CAD build for the part. Positions are in the model's coordinates, mm. Face numbers are marked on the shaded views. A direction names the side the tool comes from. Round coordinates to 2 decimals unless told otherwise and drop trailing zeros. Loops run counter-clockwise (first coordinate to the right, second up) from the corner with the lowest first, then second, coordinate; pieces in that order, holes last. Notation, with made-up numbers: M -39,-7 L -4,-7 A17 ccw -4,18 Z; hole C -29.5,-38.5 d4. An arc over 180 degrees is marked long. One line per item, written item: value. Start each with the question number.
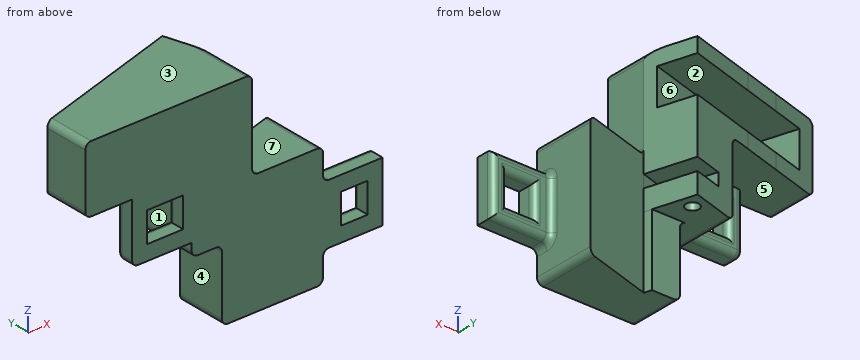
from build123d import *

# Parameters (mm, degrees)
SKETCH2_W                       = 43.976301399
SKETCH2_H                       = 37.406376753
BOSS_EXTRUDE1_DEPTH             = 3
BOSS_EXTRUDE2_REACH             = 40.151
BOSS_EXTRUDE2_DIRECTION_2_REACH = 40.151
SKETCH4_W                       = 23.72463769
SKETCH4_H                       = 6.1
CUT_EXTRUDE1_DEPTH              = 6.2
SKETCH5_W                       = 13.436339427
SKETCH5_H                       = 17.119562917
CUT_EXTRUDE2_DEPTH              = 42.11242086
CUT_EXTRUDE3_DEPTH              = 40.896849069
CUT_EXTRUDE3_DEPTH_BACK         = 40.896849069
SKETCH6_W                       = 32.063710036
SKETCH6_H                       = 2.195719192
SKETCH7_W                       = 17.859472784
SKETCH7_H                       = 24.110657561
CUT_EXTRUDE4_DEPTH              = 39.572188243
SKETCH9_W                       = 5.100000004
SKETCH9_H                       = 2.100000005
CUT_EXTRUDE5_DEPTH              = 8.272220174
SKETCH10_W                      = 4.059731886
SKETCH10_H                      = 35.210657561
CUT_EXTRUDE6_DEPTH              = 39.572188243
CUT_EXTRUDE7_DEPTH              = 11.9
SKETCH14_W                      = 10
SKETCH14_H                      = 3
BOSS_EXTRUDE3_DEPTH             = 10
SKETCH15_W                      = 4.5
SKETCH15_H                      = 5
CUT_EXTRUDE8_DEPTH              = 47.530169979
FILLET1_R                       = 1
CUT_EXTRUDE9_DEPTH              = 49.140668642
CUT_EXTRUDE10_DEPTH             = 11.9
SKETCH19_R                      = 1.1
CUT_EXTRUDE11_DEPTH             = 47.161274086
BOSS_EXTRUDE4_DEPTH             = 11.9
FILLET2_R                       = 1
SKETCH22_W                      = 10
SKETCH22_H                      = 3
BOSS_EXTRUDE5_DEPTH             = 10
SKETCH23_W                      = 6.079403202
SKETCH23_H                      = 5
CUT_EXTRUDE12_DEPTH             = 47.530169979
FILLET4_R                       = 1


with BuildPart() as part:
    # Sketch2 → Boss-Extrude1 (new body)
    with BuildSketch(Plane(origin=(0, 0, 0), x_dir=(1, 0, 0), z_dir=(0, 1, 0))):
        with Locations((6.873999922, -6.064560357)):
            Rectangle(SKETCH2_W, SKETCH2_H)
    extrude(amount=BOSS_EXTRUDE1_DEPTH)

    # Boss-Extrude2: up to this face of the body (flat: up to its plane)
    boss_extrude2_end = Plane(part.part.faces().sort_by_distance((6.873999922, 1.5, 24.767748733))[0])
    # Sketch3 → Boss-Extrude2 (add, up to the picked face)
    with BuildSketch(Plane.XY, mode=Mode.PRIVATE) as boss_extrude2_sk1:
        Polygon((3.322651848, 11.739980321), (-2.884556794, 9.919492418), (-11.054418892, 7.523385572), (-11.054418892, 3), (28.862150621, 3), (28.862150621, 10.609703324), (16.949559258, 7.115906075), (14.621493291, 15.05377326), align=None)
    boss_extrude2_tool1 = split(extrude(boss_extrude2_sk1.sketch, amount=BOSS_EXTRUDE2_REACH, mode=Mode.PRIVATE), bisect_by=boss_extrude2_end, keep=Keep.BOTH, mode=Mode.PRIVATE)
    add(boss_extrude2_tool1.solids().sort_by(Axis((9.048322, 7.098551, 0), (0, 0, 1)))[0])

    # Boss-Extrude2 direction 2: up to this face of the body (flat: up to its plane)
    boss_extrude2_direction_2_end = Plane(part.part.faces().sort_by_distance((6.873999922, 1.5, -12.63862802))[0])
    # Sketch3 → Boss-Extrude2 direction 2 (add, up to the picked face)
    with BuildSketch(Plane.XY, mode=Mode.PRIVATE) as boss_extrude2_direction_2_sk1:
        Polygon((3.322651848, 11.739980321), (-2.884556794, 9.919492418), (-11.054418892, 7.523385572), (-11.054418892, 3), (28.862150621, 3), (28.862150621, 10.609703324), (16.949559258, 7.115906075), (14.621493291, 15.05377326), align=None)
    boss_extrude2_direction_2_tool1 = split(extrude(boss_extrude2_direction_2_sk1.sketch, amount=-BOSS_EXTRUDE2_DIRECTION_2_REACH, mode=Mode.PRIVATE), bisect_by=boss_extrude2_direction_2_end, keep=Keep.BOTH, mode=Mode.PRIVATE)
    add(boss_extrude2_direction_2_tool1.solids().sort_by(Axis((9.048322, 7.098551, 0), (0, 0, -1)))[0])

    # Sketch4 → Cut-Extrude1 (cut)
    with BuildSketch(Plane(origin=(-2.907293344, 9.912824104, 0), x_dir=(0.9595812271500734, 0.2814318185656328, 0), z_dir=(-0.2814318185656328, 0.9595812271500734, 0))):
        with Locations((6.404802415, -17.022029541)):
            Rectangle(SKETCH4_W, SKETCH4_H)
    extrude(amount=-CUT_EXTRUDE1_DEPTH, mode=Mode.SUBTRACT)

    # Sketch5 → Cut-Extrude2 (cut, through all)
    with BuildSketch(Plane(origin=(-0.295587327, 0, 0), x_dir=(1, 0, 0), z_dir=(0, 1, 0))):
        with Locations((23.963316299, -16.207967274)):
            Rectangle(SKETCH5_W, SKETCH5_H)
    extrude(amount=CUT_EXTRUDE2_DEPTH, mode=Mode.SUBTRACT)

    # Sketch6 → Cut-Extrude3 (cut, two sides: drawn at the far end of the back side and taken through both)
    with BuildSketch(Plane(origin=(0, 3, 0), x_dir=(1, 0, 0), z_dir=(0, 1, 0)).offset(-CUT_EXTRUDE3_DEPTH_BACK)):
        with Locations((0.91770424, -23.669889137)):
            Rectangle(SKETCH6_W, SKETCH6_H)
    extrude(amount=CUT_EXTRUDE3_DEPTH + CUT_EXTRUDE3_DEPTH_BACK, mode=Mode.SUBTRACT)

    # Sketch7 → Cut-Extrude4 (cut, through all)
    with BuildSketch(Plane(origin=(0, 3, 0), x_dir=(1, 0, 0), z_dir=(0, 1, 0))):
        with Locations((-2.1246825, 0.583299239)):
            Rectangle(SKETCH7_W, SKETCH7_H)
    extrude(amount=CUT_EXTRUDE4_DEPTH, mode=Mode.SUBTRACT)

    # Sketch9 → Cut-Extrude5 (cut)
    with BuildSketch(Plane(origin=(-2.907293344, 9.912824104, 0), x_dir=(0.9595812271500733, 0.28143181856563293, 0), z_dir=(-0.28143181856563293, 0.9595812271500733, 0))):
        with Locations((15.995967709, -3.773090404)):
            Rectangle(SKETCH9_W, SKETCH9_H)
    extrude(amount=-CUT_EXTRUDE5_DEPTH, mode=Mode.SUBTRACT)

    # Sketch10 → Cut-Extrude6 (cut, through all)
    with BuildSketch(Plane(origin=(0, 3, 0), x_dir=(1, 0, 0), z_dir=(0, 1, 0))):
        with Locations((-13.084284835, -4.966700761)):
            Rectangle(SKETCH10_W, SKETCH10_H)
    extrude(amount=-CUT_EXTRUDE6_DEPTH, mode=Mode.SUBTRACT)

    # Sketch11 → Cut-Extrude7 (cut)
    with BuildSketch(Plane(origin=(0, 0, -12.63862802), x_dir=(-1, 0, 0), z_dir=(0, 0, -1))):
        Polygon((-6.805053892, 3), (-11.906625133, 3), (-11.906625133, 14.257540215), (-6.805053892, 12.761320373), align=None)
    extrude(amount=-CUT_EXTRUDE7_DEPTH, mode=Mode.SUBTRACT)

    # Sketch14 → Boss-Extrude3 (add)
    with BuildSketch(Plane(origin=(28.862150621, 0, 0), x_dir=(0, 0, -1), z_dir=(1, 0, 0))):
        with Locations((2.63862802, 1.5)):
            Rectangle(SKETCH14_W, SKETCH14_H)
    extrude(amount=BOSS_EXTRUDE3_DEPTH)

    # Sketch15 → Cut-Extrude8 (cut, through all)
    with BuildSketch(Plane(origin=(0, 3, 0), x_dir=(1, 0, 0), z_dir=(0, 1, 0))):
        with Locations((34.112150621, 2.63862802)):
            Rectangle(SKETCH15_W, SKETCH15_H)
    extrude(amount=-CUT_EXTRUDE8_DEPTH, mode=Mode.SUBTRACT)

    # Fillet1
    fillet1_edges = [part.edges().sort_by_distance(p)[0] for p in [
        (28.862150621, 1.5, -7.63862802),
        (28.862150621, 1.5, 2.36137198),
        (33.862150621, 3, -7.63862802),
        (38.862150621, 3, -2.63862802),
        (33.862150621, 3, 2.36137198),
        (28.862150621, 3, -2.63862802),
        (36.362150621, 3, -2.63862802),
        (34.112150621, 3, -5.13862802),
        (31.862150621, 3, -2.63862802),
        (34.112150621, 3, -0.13862802),
    ]]
    fillet(fillet1_edges, radius=FILLET1_R)

    # Sketch17 → Cut-Extrude9 (cut, through all)
    with BuildSketch(Plane(origin=(-1.914484966, 3, 0), x_dir=(1, 0, 0), z_dir=(0, 1, 0))):
        Polygon((13.8211101, 12.63862802), (13.8211101, 0.73862802), (8.719538859, 0.73862802), (8.719538859, -11.472029541), (-9.139933926, -11.472029541), (-9.139933926, 12.63862802), align=None)
    extrude(amount=-CUT_EXTRUDE9_DEPTH, mode=Mode.SUBTRACT)

    # Sketch18 → Cut-Extrude10 (cut)
    with BuildSketch(Plane(origin=(0, 0, -12.63862802), x_dir=(-1, 0, 0), z_dir=(0, 0, -1))):
        Polygon((-16.949559258, 7.115906075), (-11.906625133, 5.636883683), (-11.906625133, 14.257540215), (-14.621493291, 15.05377326), align=None)
    extrude(amount=-CUT_EXTRUDE10_DEPTH, mode=Mode.SUBTRACT)

    # Sketch19 → Cut-Extrude11 (cut, through all)
    with BuildSketch(Plane.XY.offset(2.723090401)):
        with Locations((13.083993021, 12.226100253)):
            Circle(SKETCH19_R)
    extrude(amount=-CUT_EXTRUDE11_DEPTH, mode=Mode.SUBTRACT)

    # Sketch21 → Boss-Extrude4 (add)
    with BuildSketch(Plane(origin=(0, 0, -0.73862802), x_dir=(-1, 0, 0), z_dir=(0, 0, -1))):
        Polygon((-16.949559258, 7.115906075), (-11.906625133, 5.636883683), (-11.906625133, 8.331943724), (-16.592912341, 8.331943724), align=None)
    extrude(amount=BOSS_EXTRUDE4_DEPTH)

    # Fillet2
    fillet2_edges = [part.edges().sort_by_distance(p)[0] for p in [
        (16.949559258, 3.557953038, 7.648185816),
        (16.949559258, 3.557953038, 22.572029541),
        (28.862150621, 5.304851662, 7.648185816),
        (28.862150621, 5.304851662, -12.63862802),
        (11.906625133, 4.165971862, -0.73862802),
        (11.906625133, 4.165971862, -12.63862802),
        (-11.054418892, 3.761692786, 11.472029541),
        (-11.054418892, 3.761692786, 22.572029541),
        (6.805053892, 6.380660187, -0.73862802),
        (6.805053892, 6.380660187, 11.472029541),
    ]]
    fillet(fillet2_edges, radius=FILLET2_R)

    # Sketch22 → Boss-Extrude5 (add)
    with BuildSketch(Plane(origin=(0, 0, 11.472029541), x_dir=(-1, 0, 0), z_dir=(0, 0, -1))):
        with Locations((-1.805053892, 1.5)):
            Rectangle(SKETCH22_W, SKETCH22_H)
    extrude(amount=BOSS_EXTRUDE5_DEPTH)

    # Sketch23 → Cut-Extrude12 (cut, through all)
    with BuildSketch(Plane(origin=(0, 3, 0), x_dir=(1, 0, 0), z_dir=(0, 1, 0))):
        with Locations((2.344755493, -6.472029541)):
            Rectangle(SKETCH23_W, SKETCH23_H)
    extrude(amount=-CUT_EXTRUDE12_DEPTH, mode=Mode.SUBTRACT)

    # Fillet4
    fillet4_edges = [part.edges().sort_by_distance(p)[0] for p in [
        (-3.194946108, 3, 6.472029541),
        (-3.194946108, 1.5, 1.472029541),
        (1.805053892, 3, 1.472029541),
        (5.384457094, 3, 6.472029541),
        (2.344755493, 3, 3.972029541),
        (-0.694946108, 3, 6.472029541),
        (2.344755493, 3, 8.972029541),
    ]]
    fillet(fillet4_edges, radius=FILLET4_R)


solid = part.part
(1) Mould opens along X. For the marked faces 1, 2 and 3 say: pulls with the +X half, pulls with the -X half, needs draft (parallel to the pull), parting line crosses it, or undercut.
(2) Slice it at C-C, the plane z = 19. List the corners of the cut face in (x, y), and give its area (3 significant figures).
(3) Slice it at A-A, the plane z = -4. List the corners of the cut face in (x, y).
(4) Slice it at B-B, the plane x = 13.5. List the corners of the cut face in (y, z).
(5) Probe L1, parallel to Z at x = 10, y = 9.75; L2, parallel to Z at x = 18, y = 7; L3, parallel to X at y = 4.75, z = 1.5. List the from-to ranges inside material, lowest first.
(6) Slice it at D-D, the plane x = 19. List the corners of the cut face in (y, z).
(7) Flat gauge pins, fed straight in: P1, Ø1, axis at y = 13, z = 0.5, coming from the -X side; P2, Ø3, axis at y = 4, z = -3.5, coming from the +X side; P3, Ø1.6, axis at x = 0.5, y = 0.5, coming from the -Z side. Where does each tip first touch, or does it go through?
(8) Which spindle directions (+Z, -Z, +X, -X, +Y, -Y) get a long thin tool onto all of the face, cutting with end or side? Do the marked faces 4, 5, 6 and 7. Say none if no direction does.
Check result:
1. face 1: pulls with the -X half
1. face 2: undercut
1. face 3: needs draft
2. outline: M -11.05,0 L 16.95,0 L 16.95,7.12 L 16.37,9.1 L -6.4,2.43 L -8.14,8.38 L -11.05,7.52 Z
2. area: 169 mm^2
3. outline: M 11.91,0 L 31.86,0 L 31.86,2 A1 ccw 30.86,3 L 29.86,3 A1 cw 28.86,4 L 28.86,10.61 L 16.95,7.12 L 16.59,8.33 L 11.91,8.33 Z; M 36.36,0 L 38.86,0 L 38.86,2 A1 ccw 37.86,3 L 37.36,3 A1 ccw 36.36,2 Z
4. outline: M 0,-12.64 L 8.33,-12.64 L 8.33,-0.74 L 11.21,-0.74 L 11.21,2.72 L 6.1,2.72 L 6.1,4.82 L 14.72,4.82 L 14.72,13.97 L 8.26,13.97 L 8.26,20.07 L 14.72,20.07 L 14.72,22.57 L 0,22.57 Z; M 13.24,-0.74 L 14.72,-0.74 L 14.72,2.72 L 13.24,2.72 Z
5. L1: z = -0.74 to 13.97, 20.07 to 22.57
5. L2: z = -12.64 to 7.65
5. L3: x = 6.81 to 28.86
6. outline: M 0,-12.64 L 7.72,-12.64 L 7.72,7.65 L 0,7.65 Z
7. P1: stops at x = 6.81
7. P2: stops at x = 38.73
7. P3: stops at z = 1.47
8. face 4: -Z, -X, +Y, -Y
8. face 5: -Z, -X, +Y
8. face 6: +Y
8. face 7: +Z, +X, +Y, -Y
